Check sheet for the modelled part. Datum: model origin and axes. Units: mm. Face numbers are marked on the shaded views. A direction names the side the tool comes from. Coordinates: 2 decimals unless noted, no trailing zeros. Loops run counter-clockwise (first coordinate to the right, second up) from the corner with the lowest first, then second, coordinate; pieces in that order, holes last.
```python
from build123d import *

# Parameters (mm, degrees)
F0_W      = 40
F0_H      = 40
F1_DEPTH  = 40
F2_R      = 5
F3_R      = 11
F4_DEPTH  = 7
F5_R      = 11
F6_DEPTH  = 7
F7_R      = 11
F8_DEPTH  = 7
F9_R      = 11
F10_DEPTH = 7
F11_R     = 11
F12_DEPTH = 7
F13_R     = 11
F14_DEPTH = 7
F15_R     = 10
F16_DEPTH = 2
F17_R     = 10
F18_DEPTH = 2
F19_R     = 10
F20_DEPTH = 2
F21_R     = 10
F22_DEPTH = 2
F23_R     = 10
F24_DEPTH = 2
F25_R     = 10
F26_DEPTH = 2


with BuildPart() as f1:
    # F0 (on Top) → F1 (new body)
    with BuildSketch(Plane.XY):
        with Locations((20, 20)):
            Rectangle(F0_W, F0_H)
    extrude(amount=F1_DEPTH)

    # F2
    f2_edges = [f1.edges().sort_by_distance(p)[0] for p in [
        (40, 20, 40),
        (20, 0, 40),
        (0, 0, 20),
        (40, 0, 20),
        (20, 0, 0),
        (0, 20, 40),
        (20, 40, 40),
        (40, 40, 20),
        (40, 20, 0),
        (20, 40, 0),
        (0, 40, 20),
        (0, 20, 0),
    ]]
    fillet(f2_edges, radius=F2_R)

    # F3 (on face) → F4 (cut)
    with BuildSketch(Plane.XZ):
        with Locations((20, 20)):
            Circle(F3_R)
    extrude(amount=-F4_DEPTH, mode=Mode.SUBTRACT)

    # F5 (on face) → F6 (cut)
    with BuildSketch(Plane(origin=(0, 40, 0), x_dir=(-1, 0, 0), z_dir=(0, 1, 0))):
        with Locations((-20, 20)):
            Circle(F5_R)
    extrude(amount=-F6_DEPTH, mode=Mode.SUBTRACT)

    # F7 (on face) → F8 (cut)
    with BuildSketch(Plane(origin=(0, 0, 0), x_dir=(0, -1, 0), z_dir=(-1, 0, 0))):
        with Locations((-20, 20)):
            Circle(F7_R)
    extrude(amount=-F8_DEPTH, mode=Mode.SUBTRACT)

    # F9 (on face) → F10 (cut)
    with BuildSketch(Plane.YZ.offset(40)):
        with Locations((20, 20)):
            Circle(F9_R)
    extrude(amount=-F10_DEPTH, mode=Mode.SUBTRACT)

    # F11 (on face) → F12 (cut)
    with BuildSketch(Plane(origin=(0, 0, 0), x_dir=(1, 0, 0), z_dir=(0, 0, -1))):
        with Locations((20, -20)):
            Circle(F11_R)
    extrude(amount=-F12_DEPTH, mode=Mode.SUBTRACT)

    # F13 (on face) → F14 (cut)
    with BuildSketch(Plane.XY.offset(40)):
        with Locations((20, 20)):
            Circle(F13_R)
    extrude(amount=-F14_DEPTH, mode=Mode.SUBTRACT)

    # F15 (on face) → F16 (cut)
    with BuildSketch(Plane.XY.offset(33)):
        with Locations((20, 20)):
            Circle(F15_R)
    extrude(amount=-F16_DEPTH, mode=Mode.SUBTRACT)

    # F17 (on face) → F18 (cut)
    with BuildSketch(Plane.XZ.offset(-7)):
        with Locations((20, 20)):
            Circle(F17_R)
    extrude(amount=-F18_DEPTH, mode=Mode.SUBTRACT)

    # F19 (on face) → F20 (cut)
    with BuildSketch(Plane(origin=(0, 0, 7), x_dir=(1, 0, 0), z_dir=(0, 0, -1))):
        with Locations((20, -20)):
            Circle(F19_R)
    extrude(amount=-F20_DEPTH, mode=Mode.SUBTRACT)

    # F21 (on face) → F22 (cut)
    with BuildSketch(Plane(origin=(7, 0, 0), x_dir=(0, -1, 0), z_dir=(-1, 0, 0))):
        with Locations((-20, 20)):
            Circle(F21_R)
    extrude(amount=-F22_DEPTH, mode=Mode.SUBTRACT)

    # F23 (on face) → F24 (cut)
    with BuildSketch(Plane(origin=(0, 33, 0), x_dir=(-1, 0, 0), z_dir=(0, 1, 0))):
        with Locations((-20, 20)):
            Circle(F23_R)
    extrude(amount=-F24_DEPTH, mode=Mode.SUBTRACT)

    # F25 (on face) → F26 (cut)
    with BuildSketch(Plane.YZ.offset(33)):
        with Locations((20, 20)):
            Circle(F25_R)
    extrude(amount=-F26_DEPTH, mode=Mode.SUBTRACT)


solid = f1.part
```
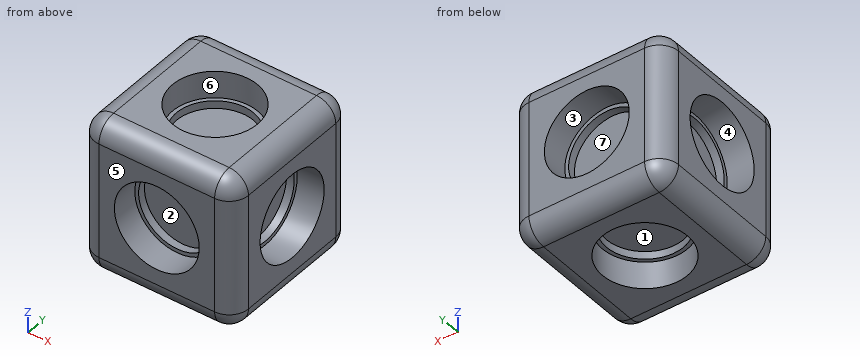
1) Depth check by flat-ended pin: pin 1 (1.5 mm diameter, centred on y = 27, z = 15.5, fed in from -X); pin 2 (17.5 mm diameter, centred on x = 20, z = 20, fed in from +Y); pin 3 (16 mm diameter, centred on x = 20, y = 20, fed in from +Z). Enter the tip coordinate at first touch or a pass-through.
Answer sheet:
pin 1: stops at x = 9
pin 2: stops at y = 31
pin 3: stops at z = 31
2) Scan lines: line 1 (Y direction, x = 20, z = 32.1); line 2 (Z direction, x = 20, y = 35). Record each from-to range of solid material in increasing order.
Answer sheet:
line 1: y = 0 to 10, 30 to 40
line 2: z = 0 to 9, 31 to 40
3) Section check A-A on z = 34. Enter the section's corners in (x, y).
Answer sheet:
outline: (0, 5) arc R5 ccw to (5, 0) - (35, 0) arc R5 ccw to (40, 5) - (40, 35) arc R5 ccw to (35, 40) - (5, 40) arc R5 ccw to (0, 35) - close; hole circle Ø22 at (20, 20)
4) Set-up check for the marked faces 1, 2 and 3: record each of +Z, -Z, +X, -X, +Y, -Y from which the full face is reachable in a straight line by a thin tool's end or side.
Answer sheet:
face 1: -Z
face 2: -Y
face 3: +Y
5) Mould release check, pull along Y, two halves, no side actions. Record for the marked faces 4, 5, 6 and 7: +Y half, -Y half, draft (parallel to the pull), parting line (faces both ways), or undercut.
Answer sheet:
face 4: undercut
face 5: -Y half
face 6: undercut
face 7: +Y half
6) Section check B-B on y = 3.5. Enter the section's corners in (x, z).
Answer sheet:
outline: (0.23, 5) arc R4.77 ccw to (5, 0.23) - (35, 0.23) arc R4.77 ccw to (39.77, 5) - (39.77, 35) arc R4.77 ccw to (35, 39.77) - (5, 39.77) arc R4.77 ccw to (0.23, 35) - close; hole circle Ø22 at (20, 20)
